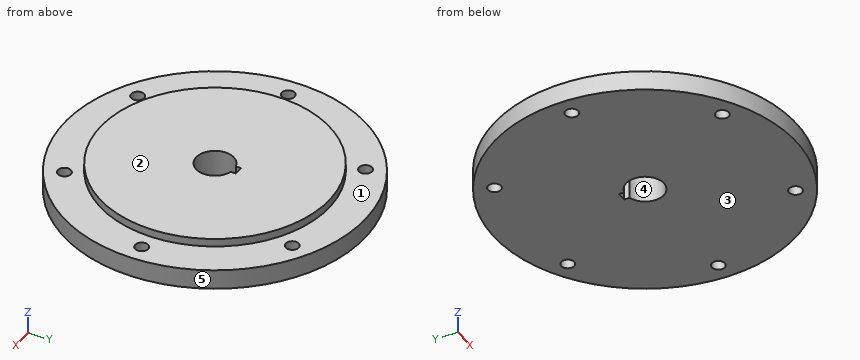
from build123d import *

# Parameters (mm, degrees)
SKETCH1_R           = 76.2
BOSS_EXTRUDE1_DEPTH = 10
SKETCH2_R           = 3.3147
CUT_EXTRUDE2_DEPTH  = 109.226059708
SKETCH4_R           = 57.9501
BOSS_EXTRUDE2_DEPTH = 4.064
SKETCH6_R           = 9.525
SKETCH6_W           = 4.7625
SKETCH6_H           = 4.7625
CUT_EXTRUDE3_DEPTH  = 109.676934517


with BuildPart() as part:
    # Sketch1 → Boss-Extrude1 (new body)
    with BuildSketch(Plane.XY):
        Circle(SKETCH1_R)
    extrude(amount=BOSS_EXTRUDE1_DEPTH)

    # Sketch2 → Cut-Extrude2 (cut, through all)
    with BuildSketch(Plane.XY):
        with Locations((66.675, 0)):
            Circle(SKETCH2_R)
        with Locations((33.3375, -57.742243797)):
            Circle(SKETCH2_R)
        with Locations((-33.3375, -57.742243797)):
            Circle(SKETCH2_R)
        with Locations((-66.675, 0)):
            Circle(SKETCH2_R)
        with Locations((-33.3375, 57.742243797)):
            Circle(SKETCH2_R)
        with Locations((33.3375, 57.742243797)):
            Circle(SKETCH2_R)
    extrude(amount=CUT_EXTRUDE2_DEPTH, mode=Mode.SUBTRACT)

    # Sketch4 → Boss-Extrude2 (add)
    with BuildSketch(Plane.XY.offset(10)):
        Circle(SKETCH4_R)
    extrude(amount=BOSS_EXTRUDE2_DEPTH)

    # Sketch6 → Cut-Extrude3 (cut, through all)
    with BuildSketch(Plane.XY.offset(14.064)):
        Circle(SKETCH6_R)
        with Locations((0, 9.525)):
            Rectangle(SKETCH6_W, SKETCH6_H)
    extrude(amount=-CUT_EXTRUDE3_DEPTH, mode=Mode.SUBTRACT)


solid = part.part
The model under review builds one solid part; all positions refer to its coordinate system, in mm. Face numbers are marked on the shaded views. A direction names the side the tool comes from. Give positions to 0.01 mm unless a question says otherwise; leave off trailing zeros. Write each loop counter-clockwise with the first axis right and the second up, starting at its lowest first coordinate (ties: lowest second). Pieces come first, ordered by that corner, then holes. Notation, with made-up numbers: M 10,28 L 29,28 A23 cw 29,67 Z; hole C -38.5,79 d5. An arc over 180 degrees is marked long. One line per question, with ' | ' between items. Start each with the question number.
Item 1: Draft analysis for pull direction X (two halves, no side actions). For the marked faces 3, 4 and 5, state which applies: released by +X, released by -X, zero draft, split by the parting line, or undercut.
Item 2: For the marked faces 1 and 2, list the 3-axis set-ups (+Z, -Z, +X, -X, +Y, -Y) from which the entire face can be reached by the end or side of a thin tool; tool diameter is ignored.
Item 3: We need section B-B on x = 0. Write out the cut boundary in (y, z) (3 decimals), plus the area to 3 significant figures.
Item 4: Wall thickness on line 1 (X direction, y = -0.5, z = 2.5); line 2 (Y direction, x = 35, z = 6.5); line 3 (X direction, y = -60, z = 7.25): over which ranges is each line inside the solid? List them lowest first. Write a range as from..to.
Item 5: We need section D-D on x = -40.5. Write out the cut boundary in (y, z).
Item 6: We need section A-A on y = 0. Write out the cut boundary in (x, z) (3 decimals), plus the area to 3 significant figures.
Item 7: We need section C-C on z = 12. Write out the cut boundary in (x, y) (3 decimals).
Item 8: For pin 1 (1 mm diameter, centred on y = 5.5, z = 9, fed in from -X); pin 2 (4 mm diameter, centred on x = 33.34, y = -57.74, fed in from -Z); pin 3 (5 mm diameter, centred on x = -0.5, z = 8, fed in from -Y); pin 4 (0.8 mm diameter, centred on y = 11, z = 9, fed in from +X), all flat-tipped, find the tip position at first contact; note any pin that passes through.
Results found:
1) face 3: zero draft | face 4: undercut | face 5: split by the parting line
2) face 1: +Z | face 2: +Z, +X, -X, +Y, -Y
3) outline: M -76.2,0 L -9.525,0 L -9.525,14.064 L -57.95,14.064 L -57.95,10 L -76.2,10 Z; M 11.906,0 L 76.2,0 L 76.2,10 L 57.95,10 L 57.95,14.064 L 11.906,14.064 Z | area: 1,690 mm2
4) line 1: x = -76.2..-69.95, -63.4..-9.51, 9.51..63.4, 69.95..76.2 | line 2: y = -67.69..-60.61, -54.87..54.87, 60.61..67.69 | line 3: x = -46.97..-35.76, -30.91..30.91, 35.76..46.97
5) outline: M -64.55,0 L 64.55,0 L 64.55,10 L 41.45,10 L 41.45,14.06 L -41.45,14.06 L -41.45,10 L -64.55,10 Z
6) outline: M -76.2,0 L -69.99,0 L -69.99,10 L -76.2,10 Z; M -63.36,0 L -9.525,0 L -9.525,14.064 L -57.95,14.064 L -57.95,10 L -63.36,10 Z; M 9.525,0 L 63.36,0 L 63.36,10 L 57.95,10 L 57.95,14.064 L 9.525,14.064 Z; M 69.99,0 L 76.2,0 L 76.2,10 L 69.99,10 Z | area: 1,590 mm2
7) outline: C 0,0 d115.9; hole M -2.381,9.223 A9.525 ccw long 2.381,9.223 L 2.381,11.906 L -2.381,11.906 Z
8) pin 1: stops at x = -76.04 | pin 2: passes through | pin 3: stops at y = -76.2 | pin 4: stops at x = 75.46
